from build123d import *

# Parameters (mm, degrees)
SKETCH_1_W          = 10
SKETCH_1_H          = 300
EXTRUDE_2_DEPTH     = 30
SKETCH_3_R          = 5
CUT_EXTRUDE_3_DEPTH = 30
SKETCH_4_R          = 5
CUT_EXTRUDE_4_DEPTH = 10


with BuildPart() as part:
    # Эскиз1 → Бобышка-Вытянуть2 (new body)
    with BuildSketch(Plane(origin=(0, 0, 0), x_dir=(1, 0, 0), z_dir=(0, 1, 0))):
        with Locations((0.774647887, -135.809859155)):
            Rectangle(SKETCH_1_W, SKETCH_1_H)
    extrude(amount=EXTRUDE_2_DEPTH)

    # Эскиз3 → Вырез-Вытянуть3 (cut)
    with BuildSketch(Plane(origin=(5.774647887, 0, 0), x_dir=(0, 0, -1), z_dir=(1, 0, 0))):
        with BuildLine():
            ThreePointArc((-0.809859155, 30), (9.797423551, 25.599339913), (14.190140845, 14.988765453))
            Line((14.190140845, 14.988765453), (14.190140845, 30))
            Line((14.190140845, 30), (-0.809859155, 30))
        make_face()
        with BuildLine():
            Line((0, 0), (14.190140845, 0))
            Line((14.190140845, 0), (14.190140845, 14.988765453))
            ThreePointArc((14.190140845, 14.988765453), (10.079887974, 4.668600871), (0, 0))
        make_face()
        with Locations((-0.821097954, 14.988765408)):
            Circle(SKETCH_3_R)
    extrude(amount=-CUT_EXTRUDE_3_DEPTH, mode=Mode.SUBTRACT)

    # Эскиз4 → Вырез-Вытянуть4 (cut)
    with BuildSketch(Plane(origin=(5.774647887, 0, 0), x_dir=(0, 0, -1), z_dir=(1, 0, 0))):
        with Locations((-255.809859155, 15)):
            Circle(SKETCH_4_R)
    extrude(amount=-CUT_EXTRUDE_4_DEPTH, mode=Mode.SUBTRACT)


solid = part.part
Build history of the part. All positions in model axes, mm. Give positions to 0.01 mm unless a question says otherwise; leave off trailing zeros. Order: outer loops, then holes, each group sorted by start corner. A loop starts at its lowest first (then second) coordinate and runs counter-clockwise, first axis right, second up. Notation, with made-up numbers: M 28,29.5 L 37,29.5 A21 ccw 37,33.5 Z; hole C -9.75,36 d3. An arc over 180 degrees is marked long. Use one line per item in the form item = value.
Q1. Wall check: probe 1 along Z at (x, y) = (-3.5, 12); probe 2 along Z at (x, y) = (1.75, 18.5); probe 3 along Z at (x, y) = (4.75, 24). Give the ranges that are in metal, low to high.
Conclusion:
probe_1 = -13.89 to -3.19, 4.83 to 251.81, 259.81 to 285.81
probe_2 = -13.77 to -2.74, 4.38 to 252.24, 259.38 to 285.81
probe_3 = -11.18 to 285.81
Q2. Slice it at A-A, the plane x = -1.5. Write the cut outline in (y, z).
Conclusion:
outline = M 0,0 A15.01 ccw 30,0.81 L 30,285.81 L 0,285.81 Z; hole C 14.99,0.82 d10; hole C 15,255.81 d10
Q3. Slice it at B-B, the plane z = 256.5. Write the cut outline in (x, y).
Conclusion:
outline = M -4.23,0 L 5.77,0 L 5.77,10.05 L -4.23,10.05 Z; M -4.23,19.95 L 5.77,19.95 L 5.77,30 L -4.23,30 Z
Q4. Pull direction Z, two halves, no side cores. Call faces 1 (the cylindrical face through (0.845, 10.108, 1.905)), 2 (the flat face through (5.775, 15, 138)), 3 (the flat face through (1, 15, 285.81)): released by +Z, released by -Z, zero draft, split by the parting line, or undercut.
Conclusion:
face_1 = undercut
face_2 = zero draft
face_3 = released by +Z
Q5. Pin check, flat tip, straight feed: P1, Ø2, axis at x = -3, y = 3, coming from the -Z side. Stop position of the tip, or through.
Conclusion:
P1 = -9.41
